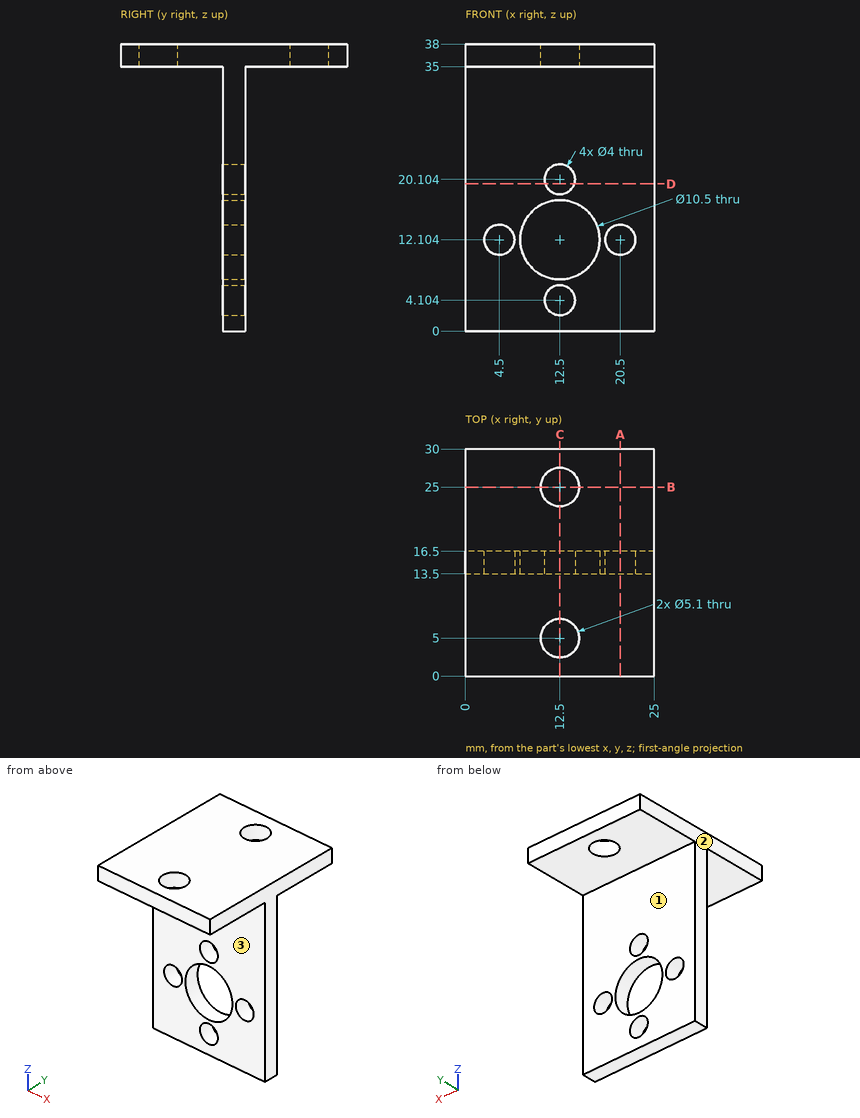
Check sheet for the drawn part. Datum: minimum x, y, z corner. Units: mm. A direction names the side the tool comes from. Round coordinates to 2 decimals unless told otherwise and drop trailing zeros. Loops run counter-clockwise (first coordinate to the right, second up) from the corner with the lowest first, then second, coordinate; pieces in that order, holes last. Notation, with made-up numbers: M 84,-2 L 101,-2 A23 ccw 101,27 Z; hole C 53,-7.5 d8. An arc over 180 degrees is marked long. One line per question, with ' | ' between items. Start each with the question number.
Item 1: Section check A-A (x = 20.5). Record the boundary of the cut face in (y, z), and give its area (3 significant figures).
Item 2: Section check B-B (y = 25). Record the boundary of the cut face in (x, z), and give its area (3 significant figures).
Item 3: Gauge pin test, flat ends, axial feed: pin 1 Ø15 at (x, y) = (8.5, 25.5) entering from -Z; pin 2 Ø12 at (x, z) = (7, 11) entering from -Y; pin 3 Ø7.5 at (x, z) = (13, 25.5) entering from +Y. Record the tip position at first contact, or that the pin passes through.
Item 4: Section check D-D (z = 19.5). Record the boundary of the cut face in (x, y), and give its area (3 significant figures).
Item 5: Section check C-C (x = 12.5). Record the boundary of the cut face in (y, z), and give its area (3 significant figures).
Item 6: Set-up check for the marked faces 1, 2 and 3: record each of +Z, -Z, +X, -X, +Y, -Y from which the full face is reachable in a straight line by a thin tool's end or side.
Item 7: Scan lines: probe 1 along Y at (x, z) = (12.5, 36.3); probe 2 along Z at (x, y) = (12.5, 15.25); probe 3 along X at (y, z) = (5, 35.75). Record each from-to range of solid material in increasing order.
Worked out:
1) outline: M 0,35 L 13.5,35 L 13.5,14.1 L 16.5,14.1 L 16.5,35 L 30,35 L 30,38 L 0,38 Z; M 13.5,0 L 16.5,0 L 16.5,10.1 L 13.5,10.1 Z | area: 183 mm^2
2) outline: M 0,35 L 9.95,35 L 9.95,38 L 0,38 Z; M 15.05,35 L 25,35 L 25,38 L 15.05,38 Z | area: 59.7 mm^2
3) pin 1: z = 35 | pin 2: y = 13.5 | pin 3: y = 16.5
4) outline: M 0,13.5 L 10.59,13.5 L 10.59,16.5 L 0,16.5 Z; M 14.41,13.5 L 25,13.5 L 25,16.5 L 14.41,16.5 Z | area: 63.6 mm^2
5) outline: M 0,35 L 2.45,35 L 2.45,38 L 0,38 Z; M 7.55,35 L 13.5,35 L 13.5,22.1 L 16.5,22.1 L 16.5,35 L 22.45,35 L 22.45,38 L 7.55,38 Z; M 13.5,0 L 16.5,0 L 16.5,2.1 L 13.5,2.1 Z; M 13.5,6.1 L 16.5,6.1 L 16.5,6.85 L 13.5,6.85 Z; M 13.5,17.35 L 16.5,17.35 L 16.5,18.1 L 13.5,18.1 Z; M 27.55,35 L 30,35 L 30,38 L 27.55,38 Z | area: 109 mm^2
6) face 1: -Z, +X, -X, +Y | face 2: +Z, -Z, -X, +Y, -Y | face 3: -Z, +X, -X, -Y
7) probe 1: 0 to 2.45, 7.55 to 22.45, 27.55 to 30 | probe 2: 0 to 2.1, 6.1 to 6.85, 17.35 to 18.1, 22.1 to 38 | probe 3: 0 to 9.95, 15.05 to 25
